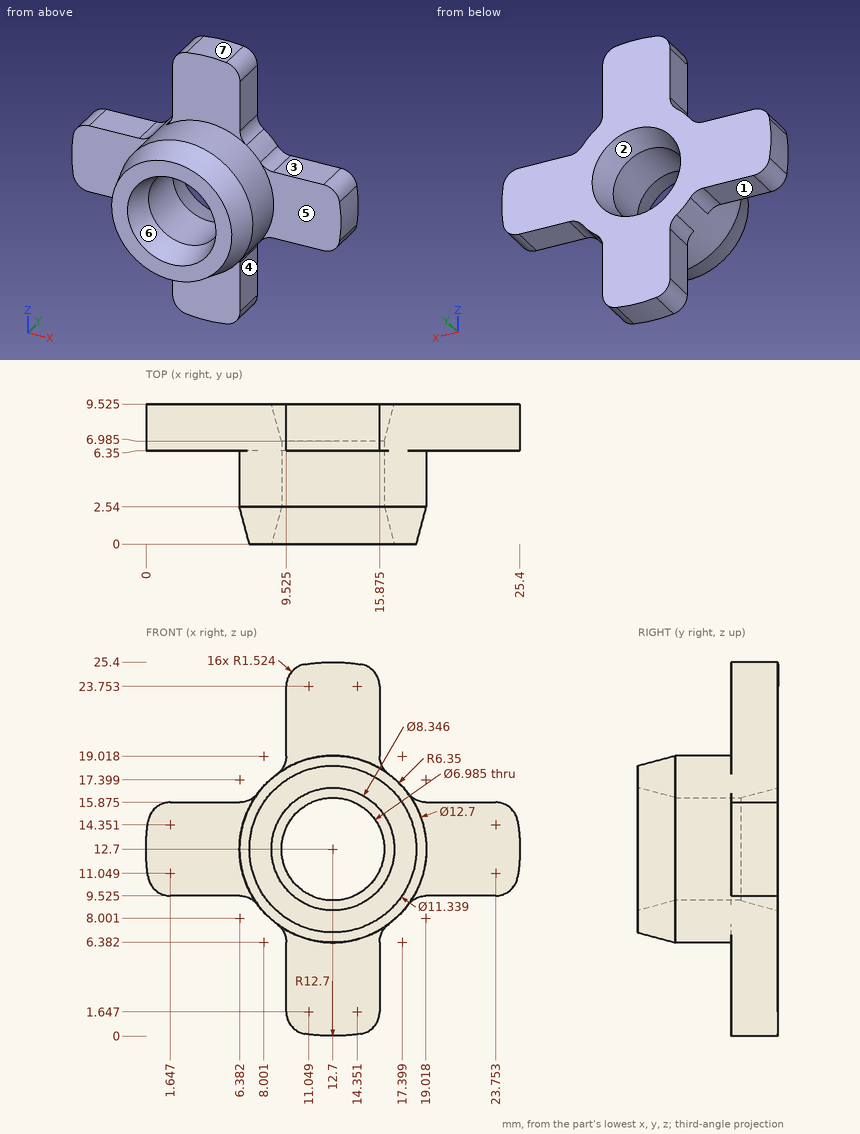
Geometry: see drawing. Coordinates: mm, zero at the bounding-box minimum. A direction names the side the tool comes from. Round coordinates to 2 decimals unless told otherwise and drop trailing zeros. Use a Markdown table: item, result. Add a question column.
1. Contact query for flat-ended pins moving along their axis: pin 1 (1 mm diameter, centred on y = 8, z = 4.5, fed in from +X) (3 decimals); pin 2 (2.5 mm diameter, centred on x = 4, y = 8.5, fed in from +Z) (3 decimals); pin 3 (1.6 mm diameter, centred on x = 4.5, y = 8, fed in from -Z) (3 decimals). Output: stop coordinate, or through.
2. Ray query, line 1 along X through (y, z) = (5, 12.7); line 2 along X through (y, z) = (7.25, 3) (1 decimal); line 3 along X through (y, z) = (1, 12) (1 decimal). Return the intervals inside material, ascending. Write a range as [from, to].
3. Set-up query: the marked faces 1, 2, 3 and 4. Return all of +Z, -Z, +X, -X, +Y, -Y with unobstructed straight access to the full face (end or side cutting, diameter ignored); none if empty.
4. Pull-direction query (Z, two-part tool) for the marked faces 5, 6 and 7; classes: +Z half, -Z half, draft (parallel to the pull), parting line (faces both ways), or undercut.
Solution:
| question | item | result |
|---|---|---|
| 1 | pin 1 | stops at x = 15.875 |
| 1 | pin 2 | stops at z = 15.875 |
| 1 | pin 3 | stops at z = 9.525 |
| 2 | line 1 | x = [6.35, 9.21], [16.19, 19.05] |
| 2 | line 2 | x = [9.5, 15.9] |
| 2 | line 3 | x = [6.8, 8.9], [16.5, 18.6] |
| 3 | face 1 | -Z, -X, +Y, -Y |
| 3 | face 2 | +Y |
| 3 | face 3 | +Z, +X, +Y, -Y |
| 3 | face 4 | -Z, +X, +Y, -Y |
| 4 | face 5 | draft |
| 4 | face 6 | undercut |
| 4 | face 7 | +Z half |
